Source: CAD feature listing. Evaluate the final solid. Frame: model axes, mm. Give positions to 0.01 mm unless a question says otherwise; leave off trailing zeros. Loops run counter-clockwise (first coordinate to the right, second up) from the corner with the lowest first, then second, coordinate; pieces in that order, holes last. Notation, with made-up numbers: (82, 49.25) -> (94, 49.25) arc R21 cw to (94, 87.25) -> close; hole circle Ø5 at (36.5, 16.25). An arc over 180 degrees is marked (long way). Return JSON: item names as keys, results as strings. Group by question number.
(1) Cut plane A-A on z = 3.45. Give the number of separate pieces and of enclosed holes in the cut face, then the cut area to 3 significant figures.
(2) Ray query, line 1 (Y direction, x = 0, z = 1.25) (3 decimals); line 2 (Y direction, x = -28, z = 1.2); line 3 (X direction, y = -29, z = 0.8). Return the intervals inside material, ascending. Write a range as from..to.
(3) Cut plane D-D on x = 29. Return loops of the section in (y, z).
(4) Cut plane B-B on x = 0. Return loops of the section in (y, z) (3 decimals), then the cut area to 3 significant figures.
(5) Pin query (flat end, axial travel): pin 1 (2 mm diameter, centred on y = 13.5, z = 1, fed in from +X); pin 2 (2 mm diameter, centred on x = 24, z = 1.5, fed in from -Y); pin 3 (4 mm diameter, centred on x = 55, y = 0, fed in from -Z); pin 4 (1.3 mm diameter, centred on x = -28, z = 3, fed in from -Y). Return the tip coordinate at first contact, or that it passes through.
```python
from build123d import *

# Parameters (mm, degrees)
ESQUISSE1_R        = 60
ESQUISSE1_R_2      = 3.5
ESQUISSE1_R_3      = 50
ESQUISSE1_R_4      = 1.595
BOSS_EXTRU_4_DEPTH = 4.5


with BuildPart() as part:
    # Esquisse1 → Boss.-Extru.4 (new body)
    # profile 1 of 2: a face of its own
    with BuildSketch(Plane.XY):
        Circle(ESQUISSE1_R)
        with Locations((-55, 0)):
            Circle(ESQUISSE1_R_2, mode=Mode.SUBTRACT)
        with Locations((55, 0)):
            Circle(ESQUISSE1_R_2, mode=Mode.SUBTRACT)
        with Locations((0, -55)):
            Circle(ESQUISSE1_R_2, mode=Mode.SUBTRACT)
        Circle(ESQUISSE1_R_3, mode=Mode.SUBTRACT)
        with Locations((0, 55)):
            Circle(ESQUISSE1_R_2, mode=Mode.SUBTRACT)
    # profile 2 of 2: a face of its own
    with BuildSketch(Plane.XY):
        with BuildLine():
            Line((5.714285714, 5.714285714), (5.714285714, 49.672396145))
            ThreePointArc((5.714285714, 49.672396145), (0, 50), (-5.714285714, 49.672396145))
            Line((-5.714285714, 49.672396145), (-5.714285714, 5.714285714))
            Line((-5.714285714, 5.714285714), (-49.672396145, 5.714285714))
            ThreePointArc((-49.672396145, 5.714285714), (-50, 0), (-49.672396145, -5.714285714))
            Line((-49.672396145, -5.714285714), (-5.714285714, -5.714285714))
            Line((-5.714285714, -5.714285714), (-5.714285714, -49.672396145))
            ThreePointArc((-5.714285714, -49.672396145), (0, -50), (5.714285714, -49.672396145))
            Line((5.714285714, -49.672396145), (5.714285714, -5.714285714))
            Line((5.714285714, -5.714285714), (49.672396145, -5.714285714))
            ThreePointArc((49.672396145, -5.714285714), (49.918031848, -2.861834443), (50, 0))
            ThreePointArc((50, 0), (49.918031848, 2.861834443), (49.672396145, 5.714285714))
            Line((49.672396145, 5.714285714), (5.714285714, 5.714285714))
        make_face()
        Circle(ESQUISSE1_R_4, mode=Mode.SUBTRACT)
    extrude(amount=BOSS_EXTRU_4_DEPTH)


solid = part.part
```
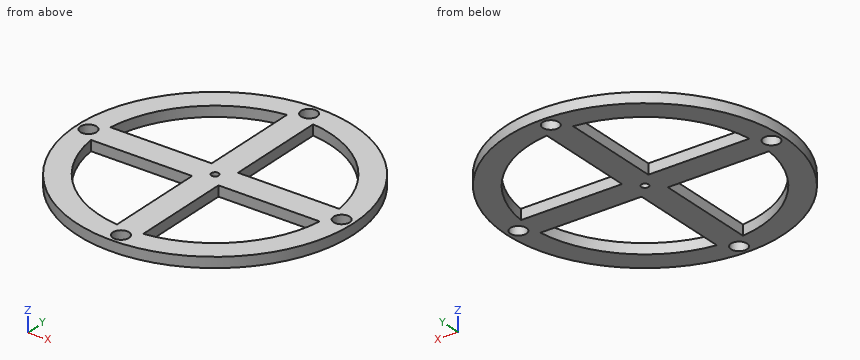
Answers:
{
 "1": {"separate pieces": "1", "enclosed holes": "9", "area": "5,440 mm²"},
 "2": {"line 1": "-60..-58.5, -51.5..-1.595, 1.595..51.5, 58.5..60", "line 2": "-53.07..-41.42, -5.71..5.71, 41.42..53.07", "line 3": "-52.53..-40.73, -5.71..5.71, 40.73..52.53"},
 "3": {"outline": "(-52.53, 0) -> (-40.73, 0) -> (-40.73, 4.5) -> (-52.53, 4.5) -> close; (-5.71, 0) -> (5.71, 0) -> (5.71, 4.5) -> (-5.71, 4.5) -> close; (40.73, 0) -> (52.53, 0) -> (52.53, 4.5) -> (40.73, 4.5) -> close"},
 "4": {"outline": "(-60, 0) -> (-58.5, 0) -> (-58.5, 4.5) -> (-60, 4.5) -> close; (-51.5, 0) -> (-1.595, 0) -> (-1.595, 4.5) -> (-51.5, 4.5) -> close; (1.595, 0) -> (51.5, 0) -> (51.5, 4.5) -> (1.595, 4.5) -> close; (58.5, 0) -> (60, 0) -> (60, 4.5) -> (58.5, 4.5) -> close", "area": "463 mm²"},
 "5": {"pin 1": "x = 58.68", "pin 2": "y = -55.42", "pin 3": "through", "pin 4": "y = -53.4"}
}
